Can you work these out from the model? Positions are in its coordinate system, mm. Coordinates: 2 decimals unless noted, no trailing zeros. Order: outer loops, then holes, each group sorted by start corner. A loop starts at its lowest first (then second) coordinate and runs counter-clockwise, first axis right, second up. Notation, with made-up numbers: (34, 76) -> (61, 76) arc R28 ccw to (61, 101) -> close; hole circle Ø11 at (20.25, -32.5). An arc over 180 degrees is marked (long way). Use a Markdown table: item, result. Add a question column.
1. Suppose I cut it at C-C, the plane x = 45. List the corners of the cut face in (y, z) for me, then the cut area to 3 significant figures.
2. Suppose I cut it at A-A, the plane x = -4. List the corners of the cut face in (y, z) for me.
3. If I drill on line 1 along Z through (x, y) = (84, 0.45); line 2 along Z through (x, y) = (44.5, 1.1); line 3 along X through (y, z) = (2.1, -75.5), over which ranges is the centre line in solid material (lowest first)? Write a range as from..to.
4. Suppose I cut it at D-D, the plane y = 1.5. State how many separate pieces and enclosed holes the cut face has, then the cut area to 3 significant figures.
5. Suppose I cut it at B-B, the plane z = -63. List the corners of the cut face in (x, y) for me, then the cut area to 3 significant figures.
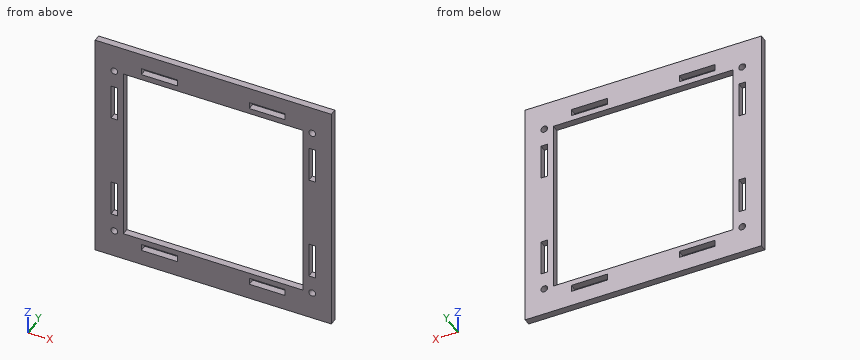
```python
from build123d import *

# Parameters (mm, degrees)
CROQUIS1_W              = 105
CROQUIS1_H              = 105
CROQUIS1_R              = 1.5
CROQUIS1_W_2            = 80
CROQUIS1_H_2            = 80
CROQUIS1_W_3            = 16
CROQUIS1_H_3            = 3
CROQUIS1_W_4            = 3
CROQUIS1_H_4            = 16
SALIENTE_EXTRUIR1_DEPTH = 3


with BuildPart() as part:
    # Croquis1 → Saliente-Extruir1 (new body)
    with BuildSketch(Plane(origin=(0, 0, 0), x_dir=(1, 0, 0), z_dir=(0, 1, 0))):
        with Locations((40, 40)):
            Rectangle(CROQUIS1_W, CROQUIS1_H)
        with Locations(Location((84, 0, 0), (0, 0, 270))):
            Circle(CROQUIS1_R, mode=Mode.SUBTRACT)
        with Locations(Location((84, 80, 0), (0, 0, 90))):
            Circle(CROQUIS1_R, mode=Mode.SUBTRACT)
        with Locations(Location((-4, 80, 0), (0, 0, 270))):
            Circle(CROQUIS1_R, mode=Mode.SUBTRACT)
        with Locations(Location((-4, 0, 0), (0, 0, 90))):
            Circle(CROQUIS1_R, mode=Mode.SUBTRACT)
        with Locations((40, 40)):
            Rectangle(CROQUIS1_W_2, CROQUIS1_H_2, mode=Mode.SUBTRACT)
        with Locations((16, -4)):
            Rectangle(CROQUIS1_W_3, CROQUIS1_H_3, mode=Mode.SUBTRACT)
        with Locations((84, 64)):
            Rectangle(CROQUIS1_W_4, CROQUIS1_H_4, mode=Mode.SUBTRACT)
        with Locations((84, 16)):
            Rectangle(CROQUIS1_W_4, CROQUIS1_H_4, mode=Mode.SUBTRACT)
        with Locations((-4, 16)):
            Rectangle(CROQUIS1_W_4, CROQUIS1_H_4, mode=Mode.SUBTRACT)
        with Locations((-4, 64)):
            Rectangle(CROQUIS1_W_4, CROQUIS1_H_4, mode=Mode.SUBTRACT)
        with Locations((64, -4)):
            Rectangle(CROQUIS1_W_3, CROQUIS1_H_3, mode=Mode.SUBTRACT)
        with Locations((64, 84)):
            Rectangle(CROQUIS1_W_3, CROQUIS1_H_3, mode=Mode.SUBTRACT)
        with Locations((16, 84)):
            Rectangle(CROQUIS1_W_3, CROQUIS1_H_3, mode=Mode.SUBTRACT)
    extrude(amount=SALIENTE_EXTRUIR1_DEPTH)


solid = part.part
```
Worked out:
| question | item | result |
|---|---|---|
| 1 | outline | (0, -92.5) -> (3, -92.5) -> (3, -80) -> (0, -80) -> close; (0, 0) -> (3, 0) -> (3, 12.5) -> (0, 12.5) -> close |
| 1 | area | 75.0 mm² |
| 2 | outline | (0, -92.5) -> (3, -92.5) -> (3, -81.5) -> (0, -81.5) -> close; (0, -78.5) -> (3, -78.5) -> (3, -72) -> (0, -72) -> close; (0, -56) -> (3, -56) -> (3, -24) -> (0, -24) -> close; (0, -8) -> (3, -8) -> (3, -1.5) -> (0, -1.5) -> close; (0, 1.5) -> (3, 1.5) -> (3, 12.5) -> (0, 12.5) -> close |
| 3 | line 1 | z = -92.5..-81.5, -78.5..-72, -56..-24, -8..-1.5, 1.5..12.5 |
| 3 | line 2 | z = -92.5..-80, 0..12.5 |
| 3 | line 3 | x = -12.5..0, 80..92.5 |
| 4 | separate pieces | 1 |
| 4 | enclosed holes | 13 |
| 4 | area | 4,210 mm² |
| 5 | outline | (-12.5, 0) -> (-5.5, 0) -> (-5.5, 3) -> (-12.5, 3) -> close; (-2.5, 0) -> (0, 0) -> (0, 3) -> (-2.5, 3) -> close; (80, 0) -> (82.5, 0) -> (82.5, 3) -> (80, 3) -> close; (85.5, 0) -> (92.5, 0) -> (92.5, 3) -> (85.5, 3) -> close |
| 5 | area | 57.0 mm² |
